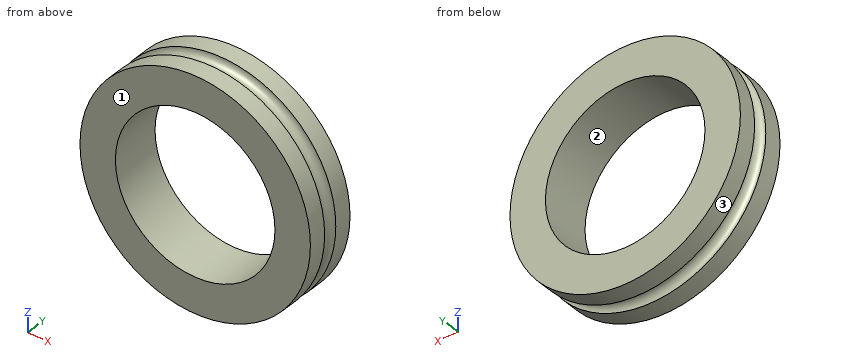
```python
from build123d import *

# Parameters (mm, degrees)
SKETCH1_R           = 15.875
BOSS_EXTRUDE1_DEPTH = 7.112
SKETCH3_R           = 10.99185
CUT_EXTRUDE1_DEPTH  = 10.16


with BuildPart() as part:
    # Sketch1 → Boss-Extrude1 (new body)
    with BuildSketch(Plane(origin=(0, 0, 0), x_dir=(1, 0, 0), z_dir=(0, 1, 0))):
        Circle(SKETCH1_R)
    extrude(amount=BOSS_EXTRUDE1_DEPTH)

    # Sketch2 → Cut-Revolve1 (revolve, cut)
    with BuildSketch(Plane.XY):
        with BuildLine():
            Line((-15.875, 4.556), (-15.875, 2.556))
            ThreePointArc((-15.875, 2.556), (-14.875, 3.556), (-15.875, 4.556))
        make_face()
    revolve(axis=Axis((0, 7.112, 0), (0, -1, 0)), mode=Mode.SUBTRACT)

    # Sketch3 → Cut-Extrude1 (cut)
    with BuildSketch(Plane(origin=(0, 7.112, 0), x_dir=(1, 0, 0), z_dir=(0, 1, 0))):
        Circle(SKETCH3_R)
    extrude(amount=-CUT_EXTRUDE1_DEPTH, mode=Mode.SUBTRACT)


solid = part.part
```
Could you check a few things on this model? Use its own coordinates, in mm. Face numbers are marked on the shaded views. Give positions to 0.01 mm unless a question says otherwise; leave off trailing zeros. Loops run counter-clockwise (first coordinate to the right, second up) from the corner with the lowest first, then second, coordinate; pieces in that order, holes last. Notation, with made-up numbers: (-12.75, 38.5) -> (38.25, 38.5) arc R16 ccw to (38.25, 48.5) -> close; hole circle Ø9 at (-21.75, 54). An arc over 180 degrees is marked (long way). Put each result on its own line as item: value.
(1) I'm going to push flat-ended pins straight in: pin 1 Ø1.5 at (x, y) = (4, 3) entering from +Z; pin 2 Ø1.5 at (y, z) = (4, 10) entering from -X; pin 3 Ø1.5 at (y, z) = (2.5, -9) entering from -X. Where does each tip first touch, or does it pass through?
Computed:
pin 1: z = 15.51
pin 2: x = -12.72
pin 3: x = -13.56
(2) Thinking about a two-plate mould opening in Z: for the marked faces 1, 2 and 3, which applies, pulls with the +Z half, pulls with the -Z half, needs draft (parallel to the pull), parting line crosses it, or undercut?
Computed:
face 1: needs draft
face 2: undercut
face 3: parting line crosses it
(3) Please list where these lines run through material, in increasing order: probe 1 along Z at (x, y) = (0, 5.5) (3 decimals); probe 2 along X at (y, z) = (0.5, 0.5); probe 3 along X at (y, z) = (6.25, 7). Write a range as [from, to].
Computed:
probe 1: [-15.875, -10.992], [10.992, 15.875]
probe 2: [-15.87, -10.98], [10.98, 15.87]
probe 3: [-14.25, -8.47], [8.47, 14.25]
(4) Imagine slicing it at A-A on x = 0. Write out the boundary of the cut face in (y, z) (3 decimals).
Computed:
outline: (0, -15.875) -> (2.556, -15.875) arc R1 cw to (4.556, -15.875) -> (7.112, -15.875) -> (7.112, -10.992) -> (0, -10.992) -> close; (0, 10.992) -> (7.112, 10.992) -> (7.112, 15.875) -> (4.556, 15.875) arc R1 cw to (2.556, 15.875) -> (0, 15.875) -> close
